Here's the drawing with two shaded views (mm, measured from the low corner). I have some questions. Round coordinates to 2 decimals unless told otherwise and drop trailing zeros. Write each loop counter-clockwise with the first axis right and the second up, starting at its lowest first coordinate (ties: lowest second). Pieces come first, ordered by that corner, then holes.
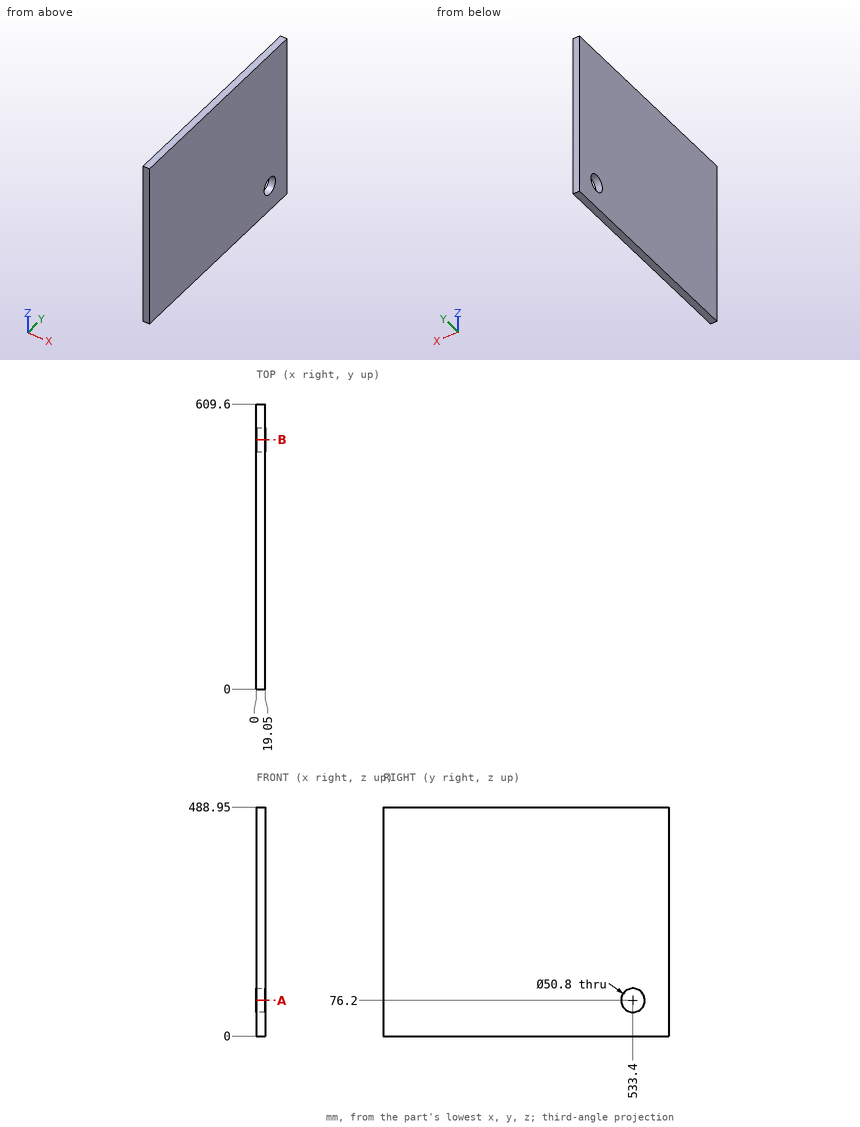
Q1. If I drill on L1, parallel to Y at x = 13.25, z = 76.2, over which ranges is the centre line in solid material (lowest first)?
Q2. Imagine slicing it at B-B, the plane y = 533.4. Write out the boundary of the cut face in (x, z), then the cut area to 3 significant figures.
Q3. Imagine slicing it at A-A, the plane z = 76.2. Write out the boundary of the cut face in (x, y), then the cut area to 3 significant figures.
Results found:
1. L1: y = 0 to 508, 558.8 to 609.6
2. outline: (0, 0) - (19.05, 0) - (19.05, 50.8) - (0, 50.8) - close; (0, 101.6) - (19.05, 101.6) - (19.05, 488.95) - (0, 488.95) - close
2. area: 8,350 mm2
3. outline: (0, 0) - (19.05, 0) - (19.05, 508) - (0, 508) - close; (0, 558.8) - (19.05, 558.8) - (19.05, 609.6) - (0, 609.6) - close
3. area: 10,600 mm2
